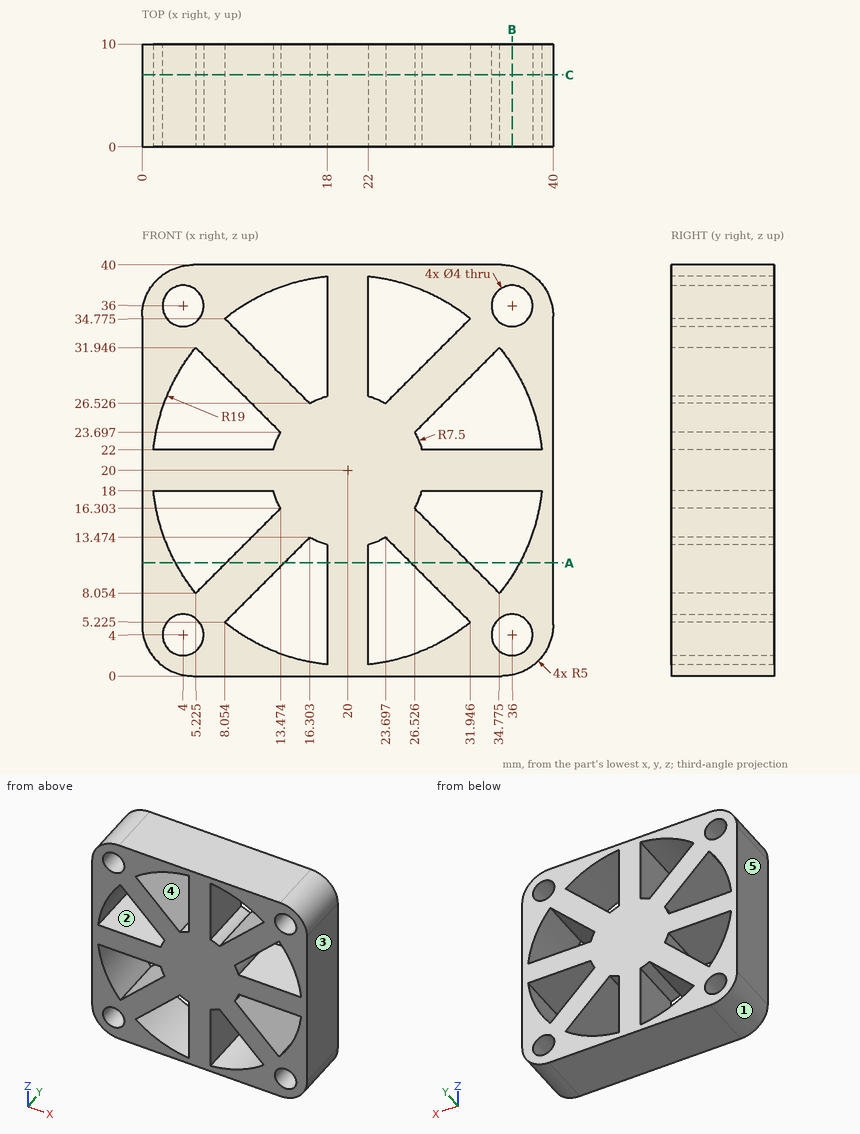
Design review of the part shown in the three views and the two pictorial views. Dimensions are in mm from the part's minimum x, y and z. A direction names the side the tool comes from. Give positions to 0.01 mm unless a question says otherwise; leave off trailing zeros. Write each loop counter-clockwise with the first axis right and the second up, starting at its lowest first coordinate (ties: lowest second). Pieces come first, ordered by that corner, then holes.
Item 1: The part is to be moulded in two halves that separate along X. For the marked faces 1, 2 and 3, say which applies: +X half, -X half, draft (parallel to the pull), parting line (faces both ways), or undercut.
Item 2: Insertion check: P1, Ø5, axis at x = 36, z = 4, coming from the -Y side. The pin has a flat end and moves straight along its axis. Give the tip position at first contact, or say it passes through.
Item 3: Take a section at C-C (y = 7). Give the number of separate pieces and of enclosed holes in the cut face.
Item 4: Machinability: for the marked faces 4 and 5, which of the approach directions +Z, -Z, +X, -X, +Y, -Y give a long, thin tool a straight path to every point of the face, cutting with its end or side? Answer none if there is none.
Item 5: Take a section at A-A (z = 11). Give the boundary of the cut face in (x, y).
Item 6: Wall thickness on probe 1 along Z at (x, y) = (11.5, 1) (1 decimal); probe 2 along X at (y, z) = (8.25, 24) (1 decimal); probe 3 along Z at (x, y) = (33, 8.75): over which ranges is each line inside the solid? List them lowest first.
Item 7: Take a section at B-B (x = 36). Give the boundary of the cut face in (y, z).
Established:
1. face 1: -X half
1. face 2: undercut
1. face 3: +X half
2. P1: stops at y = 0
3. separate pieces: 1
3. enclosed holes: 12
4. face 4: +Y, -Y
4. face 5: +Z, -Z, -X, +Y, -Y
5. outline: (0, 0) - (3.27, 0) - (3.27, 10) - (0, 10) - close; (8.17, 0) - (13.83, 0) - (13.83, 10) - (8.17, 10) - close; (18, 0) - (22, 0) - (22, 10) - (18, 10) - close; (26.17, 0) - (31.83, 0) - (31.83, 10) - (26.17, 10) - close; (36.73, 0) - (40, 0) - (40, 10) - (36.73, 10) - close
6. probe 1: z = 0 to 3, 8.7 to 14.3, 18 to 22, 25.7 to 31.3, 37 to 40
6. probe 2: x = 0 to 1.4, 13.2 to 26.8, 38.6 to 40
6. probe 3: z = 0 to 9.83, 18 to 22, 30.17 to 40
7. outline: (0, 0.1) - (10, 0.1) - (10, 2) - (0, 2) - close; (0, 6) - (10, 6) - (10, 9.75) - (0, 9.75) - close; (0, 18) - (10, 18) - (10, 22) - (0, 22) - close; (0, 30.25) - (10, 30.25) - (10, 34) - (0, 34) - close; (0, 38) - (10, 38) - (10, 39.9) - (0, 39.9) - close
